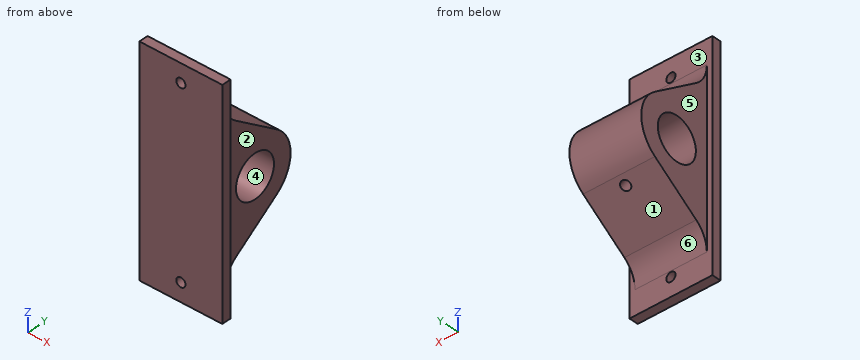
Autodesk Inventor part; units mm, degrees
ref_plane "YZ Plane" through (0, 0, 0) normal (1, 0, 0) x (0, 1, 0)
ref_plane "XZ Plane" through (0, 0, 0) normal (0, 1, 0) x (-1, 0, 0)
ref_plane "XY Plane" through (0, 0, 0) normal (0, 0, 1) x (1, 0, 0)
sketch "Sketch6" plane through (0, 0, 0) normal (0, 1, 0) x (-1, 0, 0)
  line L0 (22.5, 0) -> (22.5, -60)
  line L1 (22.5, -60) -> (-22.5, -60)
  line L2 (-22.5, -60) -> (-22.5, 0)
  circle A0 centre (0, -50) radius 2.5
  line L3 (-22.5, 0) -> (22.5, 0)
  point P0 (0, 0)
  dimension "d85" = 22.5
  dimension "d86" = 60
  dimension "d87" = 45
  dimension "d89" = 5
extrude "Extrusion3" add sketch "Sketch6" along normal blind 5
mirror "Mirror3" about plane through (-22.5, 0, 0) normal (0, 0, 1) of "Extrusion3"
sketch "Sketch7" plane through (0, 0, -60) normal (1, 0, 0) x (0, 0, -1)
  arc A0 (-43.7585, 36.671) -> (-76.2415, 36.671) centre (-60, 25) ccw
  circle A1 centre (-60, 23.3) radius 11.6
  line L0 (0, 5) -> (-120, 5)
  line L1 (-60, 5) -> (-99, 5)
  line L2 (-99, 5) -> (-76.2415, 36.671)
  line L3 (-60, 5) -> (-21, 5)
  line L4 (-21, 5) -> (-43.7585, 36.671)
  line L5 (-21, 5) -> (-99, 5)
  line L6 (-60, 17.6583) -> (-60, 50) construction
  line L7 (-120, 0) -> (0, 0)
  point P0 (-60, 0)
  point P1 (-60, 0)
  point P2 (-60, 0)
  dimension "d92" = 40
  dimension "d93" = 23.2
  dimension "d94" = 39
  dimension "d95" = 39
  dimension "d104" = 23.3
  dimension "d105" = 25
extrude "Extrusion6" add sketch "Sketch7" along normal mid plane 39
sketch "Sketch10" plane through (19.5, 0, -60) normal (1, 0, 0) x (0, 0, -1)
  circle A0 centre (-60, 23.3) radius 11.6 construction
  point P0 (-60, 0)
hole "Hole4" at (19.5, 23.3, 0) direction (-1, 0, 0) diameter 22.25 depth 7
sketch "Sketch11" plane through (-19.5, 0, -60) normal (-1, 0, 0) x (0, 0, 1)
  circle A0 centre (60, 23.3) radius 11.6
  point P0 (60, 0)
hole "Hole5" at (-19.5, 23.3, 0) at (-19.5, 23.3, 0) direction (1, 0, 0) diameter 22.3 depth 7
fillet "Fillet1" radius 15.5 2 edges at (0, 5, 39) (0, 5, -39)
sketch "Sketch12" plane through (19.5, 36.671, -16.2415) normal (0, 0.5835502, -0.812077) x (-1, 0, 0)
  circle A0 centre (19.5, -5) radius 2.5
  point P0 (19.5, -20.3019)
  dimension "d121" = 5
extrude "Extrusion7" cut sketch "Sketch12" against normal blind 28.75
properties part number "8P - MainWing Joint"
Geometry: final body of the model. Coordinates: model frame, mm. Face numbers are marked on the shaded views. A direction names the side the tool comes from. Coordinates: 2 decimals unless noted, no trailing zeros. Loops run counter-clockwise (first coordinate to the right, second up) from the corner with the lowest first, then second, coordinate; pieces in that order, holes last. Notation, with made-up numbers: M 1.25,70.25 L 48.25,70.25 A24 ccw 48.25,93.25 Z; hole C -28.5,82 d3. An arc over 180 degrees is marked long. One line per item, written item: value. Start each with the question number.
1) Pin query (flat end, axial travel): P1, Ø10, axis at x = -16, z = 14.5, coming from the +Y side; P2, Ø8, axis at x = -17.5, y = 13, coming from the -Z side; P3, Ø8, axis at x = 4, z = -27.5, coming from the +Y side. Return the tip coordinate at first contact, or that it passes through.
2) Cut plane B-B (x = 10.5). Return loops of the section in (y, z).
3) Cut plane C-C (z = 0). Return loops of the section in (x, y).
4) Cut plane D-D (x = 0). Return loops of the section in (y, z).
5) Material intervals for L1, parallel to Z at x = 0, y = 3; L2, parallel to X at y = 3, z = 50; L3, parallel to Y at x = 4, z = -54, sorted ascending. Write a range as from..to.
6) Draft query along Y for the marked faces 4, 5 and 6. Return one class per face: released by +Y, released by -Y, zero draft, split by the parting line, or undercut.
7) Cut plane A-A (z = 50). Return loops of the section in (x, y).
8) Reachability of the marked faces 1, 2 and 3 from +Z, -Z, +X, -X, +Y, -Y: full face, straight path, thin tool, end or side. Return the list, or none.
Evaluation:
1. P1: y = 42.6
1. P2: z = -36.56
1. P3: y = 26.57
2. outline: M 0,-60 L 5,-60 L 5,-46.95 A15.5 cw 11.45,-34.36 L 36.67,-16.24 A20 ccw 36.67,16.24 L 11.45,34.36 A15.5 cw 5,46.95 L 5,60 L 0,60 Z; hole C 23.3,0 d23.2
3. outline: M -22.5,0 L 22.5,0 L 22.5,5 L 19.5,5 L 19.5,11.7 L -19.5,11.7 L -19.5,5 L -22.5,5 Z; M -19.5,34.9 L 19.5,34.9 L 19.5,45 L -19.5,45 Z
4. outline: M 0,-60 L 5,-60 L 5,-52.5 L 0,-52.5 Z; M 0,-47.5 L 5,-47.5 L 5,-46.95 A15.5 cw 11.45,-34.36 L 30.58,-20.62 L 24.08,-11.57 A11.6 cw long 29.13,-10.03 L 34.64,-17.7 L 36.67,-16.24 A20 ccw 36.67,16.24 L 11.45,34.36 A15.5 cw 5,46.95 L 5,47.5 L 0,47.5 Z; M 0,52.5 L 5,52.5 L 5,60 L 0,60 Z
5. L1: -60..-52.5, -47.5..47.5, 52.5..60
5. L2: -22.5..-2.5, 2.5..22.5
5. L3: 0..5
6. face 4: undercut
6. face 5: zero draft
6. face 6: released by +Y
7. outline: M -22.5,0 L -2.5,0 L -2.5,5 L -22.5,5 Z; M 2.5,0 L 22.5,0 L 22.5,5 L 2.5,5 Z
8. face 1: -Z, +X, -X, +Y
8. face 2: +Z, -Z, +X, +Y
8. face 3: +Y
